Could you check a few things on this model? Use its own coordinates, in mm. A direction names the side the tool comes from. Give positions to 0.01 mm unless a question says otherwise; leave off trailing zeros. Loops run counter-clockwise (first coordinate to the right, second up) from the corner with the lowest first, then second, coordinate; pieces in that order, holes last. Notation, with made-up numbers: (58.5, -28.75) -> (96.5, -28.75) arc R20 ccw to (96.5, -3.75) -> close; hole circle Ø5 at (-23.75, 31). An arc over 180 degrees is marked (long way). Put each result on its own line as item: value.
```python
from build123d import *

# Parameters (mm, degrees)
SKETCH_1_R               = 23.5
EXTRUDE_1_DEPTH          = 5
SKETCH_2_R               = 1.55
CUT_EXTRUDE_1_DEPTH      = 10
PATTERN_CIRCULAR_1_COUNT = 6
SKETCH_3_R               = 1.55
CUT_EXTRUDE_2_DEPTH      = 10
SKETCH_4_R               = 4
SKETCH_4_R_2             = 1.5
EXTRUDE_2_DEPTH          = 4
PATTERN_CIRCULAR_2_COUNT = 6


with BuildPart() as part:
    # 草图1 → 凸台-拉伸1 (new, symmetric)
    with BuildSketch(Plane.XY):
        with BuildLine():
            ThreePointArc((-44.047161963, -22.216294005), (-27, 0), (-44.047161963, 22.216294005))
            ThreePointArc((-44.047161963, 22.216294005), (-45.963802781, 23.89714289), (-45.797072706, 26.440952255))
            ThreePointArc((-45.797072706, 26.440952255), (-43.677434211, 27.857249418), (-41.263455967, 27.037814222))
            ThreePointArc((-41.263455967, 27.037814222), (-13.5, 23.382685902), (-2.783705995, 49.254108227))
            ThreePointArc((-2.783705995, 49.254108227), (-2.28636857, 51.754392308), (0, 52.88190451))
            ThreePointArc((0, 52.88190451), (2.28636857, 51.754392308), (2.783705995, 49.254108227))
            ThreePointArc((2.783705995, 49.254108227), (13.5, 23.382685902), (41.263455967, 27.037814222))
            ThreePointArc((41.263455967, 27.037814222), (43.677434211, 27.857249418), (45.797072706, 26.440952255))
            ThreePointArc((45.797072706, 26.440952255), (45.963802781, 23.89714289), (44.047161963, 22.216294005))
            ThreePointArc((44.047161963, 22.216294005), (27, 0), (44.047161963, -22.216294005))
            ThreePointArc((44.047161963, -22.216294005), (45.963802781, -23.89714289), (45.797072706, -26.440952255))
            ThreePointArc((45.797072706, -26.440952255), (43.677434211, -27.857249418), (41.263455967, -27.037814222))
            ThreePointArc((41.263455967, -27.037814222), (13.5, -23.382685902), (2.783705995, -49.254108227))
            ThreePointArc((2.783705995, -49.254108227), (2.28636857, -51.754392308), (0, -52.88190451))
            ThreePointArc((0, -52.88190451), (-2.28636857, -51.754392308), (-2.783705995, -49.254108227))
            ThreePointArc((-2.783705995, -49.254108227), (-13.5, -23.382685902), (-41.263455967, -27.037814222))
            ThreePointArc((-41.263455967, -27.037814222), (-43.677434211, -27.857249418), (-45.797072706, -26.440952255))
            ThreePointArc((-45.797072706, -26.440952255), (-45.963802781, -23.89714289), (-44.047161963, -22.216294005))
        make_face()
        Circle(SKETCH_1_R, mode=Mode.SUBTRACT)
    extrude(amount=EXTRUDE_1_DEPTH, both=True)

    # 草图2 → 切除-拉伸1 (cut)
    with BuildSketch(Plane.XY.offset(5)):
        with Locations((0, 50)):
            Circle(SKETCH_2_R)
    cut_extrude_1 = extrude(amount=-CUT_EXTRUDE_1_DEPTH, mode=Mode.SUBTRACT)

    # 阵列(圆周)1: 切除-拉伸1 ×6 about axis
    pattern_circular_1_axis = Axis((0, 0, 0), (0, 0, 1))
    for i in range(1, PATTERN_CIRCULAR_1_COUNT):
        add(cut_extrude_1.rotate(pattern_circular_1_axis, i * 360 / PATTERN_CIRCULAR_1_COUNT), mode=Mode.SUBTRACT)

    # 草图3 → 切除-拉伸2 (cut)
    with BuildSketch(Plane.XY.offset(5)):
        with Locations((0, 27.5)):
            Circle(SKETCH_3_R)
        with Locations((23.815698604, 13.75)):
            Circle(SKETCH_3_R)
        with Locations((23.815698604, -13.75)):
            Circle(SKETCH_3_R)
        with Locations((0, -27.5)):
            Circle(SKETCH_3_R)
        with Locations((-23.815698604, -13.75)):
            Circle(SKETCH_3_R)
        with Locations((-23.815698604, 13.75)):
            Circle(SKETCH_3_R)
    extrude(amount=-CUT_EXTRUDE_2_DEPTH, mode=Mode.SUBTRACT)

    # 草图4 → 凸台-拉伸2 (add)
    with BuildSketch(Plane(origin=(0, 0, -5), x_dir=(-1, 0, 0), z_dir=(0, 0, -1))):
        with Locations(Location((-43.301270189, 25, 0), (0, 0, 295.743562627))):
            Circle(SKETCH_4_R)
        with Locations((-43.301270189, 25)):
            Circle(SKETCH_4_R_2, mode=Mode.SUBTRACT)
    extrude_2 = extrude(amount=EXTRUDE_2_DEPTH)

    # 阵列(圆周)2: 凸台-拉伸2 ×6 about axis
    pattern_circular_2_axis = Axis((0, 0, 0), (0, 0, 1))
    for i in range(1, PATTERN_CIRCULAR_2_COUNT):
        add(extrude_2.rotate(pattern_circular_2_axis, i * 360 / PATTERN_CIRCULAR_2_COUNT))


solid = part.part
```
1. Thinking about a two-plate mould opening in Y: for faces 4 (the face through (-41.6, 25.1, -9)), 5 (the face through (1.577, -46.324, -6.972)), which applies, pulls with the +Y half, pulls with the -Y half, needs draft (parallel to the pull), parting line crosses it, or undercut?
Recorded:
face 4: needs draft
face 5: undercut
2. If we section it at C-C (z = 1.25): Count the separate pieces of the cut face and the enclosed holes in it, then the cut area to 3 significant figures.
Recorded:
separate pieces: 1
enclosed holes: 13
area: 1,610 mm^2
3. If we section it at B-B (y = -13.75): List the corners of the cut face in (x, z) for me.
Recorded:
outline: (-31.56, -5) -> (-25.37, -5) -> (-25.37, 5) -> (-31.56, 5) -> close; (-22.27, -5) -> (-19.06, -5) -> (-19.06, 5) -> (-22.27, 5) -> close; (19.06, -5) -> (22.27, -5) -> (22.27, 5) -> (19.06, 5) -> close; (25.37, -5) -> (31.56, -5) -> (31.56, 5) -> (25.37, 5) -> close
4. For faces 1 (the face through (-22.34, 14.22, 0.07)), 2 (the face through (46.65, -27.19, -6.97)), 3 (the face through (46, 27, -5)), which set-ups out of +Z, -Z, +X, -X, +Y, -Y let a thin tool reach every point of the face, with its end or its side?
Recorded:
face 1: +Z, -Z
face 2: -Z
face 3: +Z
5. If we section it at A-A (x = -30.5): List the corners of the cut face in (y, z) for me, then the cut area to 3 significant figures.
Recorded:
outline: (-20.97, -5) -> (-12.2, -5) -> (-12.2, 5) -> (-20.97, 5) -> close; (12.2, -5) -> (20.97, -5) -> (20.97, 5) -> (12.2, 5) -> close
area: 175 mm^2
6. I'm going to push flat-ended pins straight in: pin 1 (6 mm diameter, centred on y = -14.5, z = 2, fed in from -X); pin 2 (2 mm diameter, centred on x = 37, y = 25, fed in from -Z); pin 3 (6 mm diameter, centred on y = 31, z = -1.5, fed in from +X); pin 4 (5 mm diameter, centred on y = -13, z = -5.5, fed in from +X). Where does each tip first touch, or does it pass through?
Recorded:
pin 1: stops at x = -35.08
pin 2: passes through
pin 3: stops at x = 7.83
pin 4: stops at x = 32.96
7. If we section it at D-D (y = 40.5): List the corners of the cut face in (x, z) for me, then the cut area to 3 significant figures.
Recorded:
outline: (-2.17, -5) -> (2.17, -5) -> (2.17, 5) -> (-2.17, 5) -> close
area: 43.4 mm^2
8. I need wall thicknesses on line 1 (Y direction, x = 0, z = -6.55); line 2 (Y direction, x = -25, z = 2); line 3 (X direction, y = 24.5, z = -5.5). Which ranges of each line are inside material? Lowest first, please.
Recorded:
line 1: y = -54 to -51.5, -48.5 to -46, 46 to 48.5, 51.5 to 54
line 2: y = -20.3 to -14.75, -12.75 to 12.75, 14.75 to 20.3
line 3: x = -47.27 to -44.72, -41.89 to -39.33, 39.33 to 41.89, 44.72 to 47.27
